Read the model definition and answer for the solid it produces. Units are mm, in the model's axes. Give positions to 0.01 mm unless a question says otherwise; leave off trailing zeros. Loops run counter-clockwise (first coordinate to the right, second up) from the corner with the lowest first, then second, coordinate; pieces in that order, holes last.
(1) Straight lines are drawn through the part: probe 1 along X at (y, z) = (-0.65, 29); probe 2 along X at (y, z) = (-0.65, 37); probe 3 along Z at (x, y) = (33.5, -0.65). For each, find the intervals that lie inside material, in ascending order.
(2) Each of these flat-tipped pins is pushed along its axis until it touches: P1, Ø0.5, axis at x = -1, y = -0.5, coming from the -Z side; P2, Ø0.5, axis at y = -0.5, z = -6.5, coming from the +X side; P3, Ø0.6, axis at y = -0.5, z = -5.5, coming from the +X side. Where does it stop, or does it pass through?
(3) Find section B-B, the plane z = -30. Write down the section's boundary in (x, y).
(4) Find section A-A, the plane x = 36.5. Write down the section's boundary in (y, z).
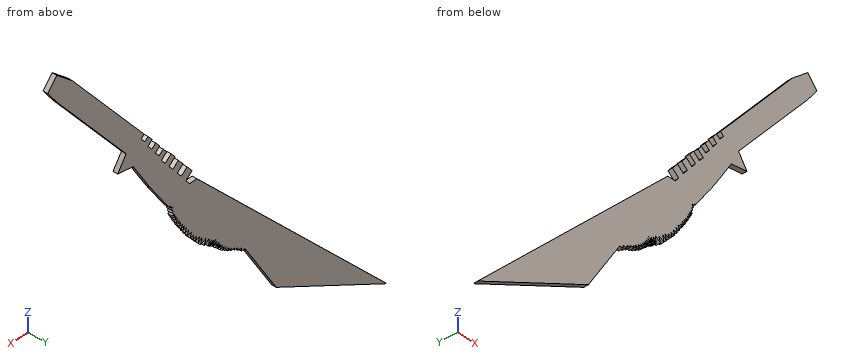
```python
from build123d import *

# Parameters (mm, degrees)
F1_DEPTH = 1.27


with BuildPart() as f1:
    # F0 (on Front) → F1 (new body)
    with BuildSketch(Plane.XZ):
        Polygon((31.435996, 36.724295), (51.609881, 61.207164), (54.505855, 65.174182), (51.805742, 68.258226), (47.221687, 64.244838), (27.331568, 40.106345), align=None)
        Polygon((33.907399, 33.032119), (31.435996, 36.724295), (27.331568, 40.106345), (26.134862, 38.654033), (27.016983, 37.927165), (25.923324, 36.599909), (24.968057, 37.387049), (23.803444, 35.973684), (24.991162, 34.882604), (23.87859, 33.532396), (22.737729, 34.472465), (21.549792, 33.030793), (22.830821, 31.975225), (21.737482, 30.648356), (20.536821, 31.637701), (19.501161, 30.380832), (21.054899, 29.100551), (19.916793, 27.719354), (18.198055, 29.135594), (17.023039, 27.709604), (18.789157, 26.254323), (17.689198, 24.919421), (16.074062, 26.250293), (14.70201, 24.585181), (16.381021, 23.201676), (15.179227, 21.743188), (13.492946, 23.132684), (11.994152, 21.313759), (13.842246, 19.79093), (12.76418, 18.482599), (10.629401, 18.482599), (-45.317493, -40.18655), (-12.743622, -22.388158), (-4.106611, -8.254142), (-3.546211, -7.337077), (-2.509889, -7.337077), (-2.509889, -6.584582), (-1.465608, -6.584582), (-1.465608, -5.911632), (-0.487286, -5.911632), (-0.487286, -5.406398), (0.678638, -5.406398), (0.294408, -4.989546), (1.541625, -4.989546), (0.918016, -4.439303), (2.38533, -4.439303), (1.798405, -3.852378), (3.265719, -3.852378), (2.458696, -3.302135), (3.92601, -3.302135), (3.082028, -2.731179), (4.379619, -2.731179), (3.326856, -2.339453), (4.89376, -2.339453), (3.722346, -1.922547), (5.389937, -1.922547), (4.072334, -1.366683), (5.822276, -1.366683), (4.475968, -0.654733), (6.313379, -1.099426), (4.857528, 0), (6.717285, -0.830613), (5.429589, 0.337804), (6.98239, -0.678996), (6.13036, 0.893481), (7.173772, -0.558674), (6.974065, 1.296992), (8.441378, 0.343238), (7.964502, 1.847235), (9.538486, 1.173172), (9.024926, 2.787217), (10.272143, 1.980195), (9.758583, 3.447509), (11.079165, 2.933949), (10.74902, 3.997752), (11.77614, 3.740972), (11.519359, 4.804774), (12.54648, 4.584677), (12.253017, 5.795211), (13.426868, 5.795211), (13.023357, 6.859014), (14.123842, 6.859014), (13.646965, 7.886133), (14.784134, 7.886133), (14.270574, 8.619791), (15.297693, 8.583108), (14.784134, 9.390131), (15.811253, 9.390131), (15.297693, 10.178116), (16.224287, 10.178116), (15.719054, 10.838806), (16.690658, 10.838806), (16.34088, 11.732681), (17.118163, 11.732681), (16.651792, 12.471099), (17.506804, 12.471099), (17.001571, 13.099144), (17.774189, 13.099144), (17.401093, 13.596605), (17.954518, 14.011674), (17.614069, 14.465607), (18.167494, 14.880675), (17.701125, 15.502501), (18.400678, 15.502501), (18.400678, 16.024083), (18.874273, 16.024083), (24.364635, 24.158362), (29.332101, 32.292642), align=None)
    extrude(amount=F1_DEPTH)


solid = f1.part
```
Entries:
1. probe 1: x = 18.09 to 18.36, 20.97 to 27.32
1. probe 2: x = 24.65 to 25.44, 26.25 to 31.66
1. probe 3: z = 32.97 to 33.64, 39.23 to 47.59
2. P1: stops at z = -5.91
2. P2: stops at x = -1.47
2. P3: stops at x = 0.68
3. outline: (-35.6, -1.27) - (-26.67, -1.27) - (-26.67, 0) - (-35.6, 0) - close
4. outline: (-1.27, 42.87) - (0, 42.87) - (0, 51.23) - (-1.27, 51.23) - close
